The model under review builds one solid part; all positions refer to its coordinate system, in mm. A direction names the side the tool comes from. Coordinates: 2 decimals unless noted, no trailing zeros. Loops run counter-clockwise (first coordinate to the right, second up) from the corner with the lowest first, then second, coordinate; pieces in that order, holes last. Notation, with made-up numbers: M 15.5,-24.75 L 25.5,-24.75 A25 ccw 25.5,12.25 Z; hole C 62,-19 d10. An arc over 180 degrees is marked long. One line per item, written item: value.
```python
from build123d import *

# Parameters (mm, degrees)
SKICA2_W                 = 95
SKICA2_H                 = 50
SKICA2_W_2               = 92.6
SKICA2_H_2               = 47.6
P_IDAT_VYSUNUT_M3_DEPTH  = 11
SKICA7_R                 = 1.2
SKICA7_W                 = 11
SKICA7_H                 = 6.3
ODEBRAT_VYSUNUT_M1_DEPTH = 71.924466864
SKICA8_R                 = 2.65
SKICA8_W                 = 15.4
SKICA8_H                 = 7.7
ODEBRAT_VYSUNUT_M2_DEPTH = 71.924466864
SKICA9_R                 = 3.15
ODEBRAT_VYSUNUT_M3_DEPTH = 15
SKICA12_W                = 95
SKICA12_H                = 50
P_IDAT_VYSUNUT_M4_DEPTH  = 1.2
SKICA13_R                = 8
SKICA13_W                = 22
SKICA13_H                = 25
SKICA13_R_2              = 1.2
SKICA13_R_3              = 1.25
ODEBRAT_VYSUNUT_M4_DEPTH = 1.2


with BuildPart() as part:
    # Skica2 → Přidat vysunutím3 (new body)
    with BuildSketch(Plane.XY.offset(1.2)):
        with Locations((47.5, -25)):
            Rectangle(SKICA2_W, SKICA2_H)
        with Locations((47.5, -25)):
            Rectangle(SKICA2_W_2, SKICA2_H_2, mode=Mode.SUBTRACT)
    extrude(amount=P_IDAT_VYSUNUT_M3_DEPTH)

    # Skica7 → Odebrat vysunutím1 (cut, through all)
    with BuildSketch(Plane(origin=(45, -1.2, 0), x_dir=(1, 0, 0), z_dir=(0, -1, 0))):
        with Locations(Location((-20.9, 6.35, 0), (0, 0, 270))):
            Circle(SKICA7_R)
        with Locations(Location((-5.7, 6.35, 0), (0, 0, 270))):
            Circle(SKICA7_R)
        with Locations((-13.3, 6.35)):
            Rectangle(SKICA7_W, SKICA7_H)
    extrude(amount=-ODEBRAT_VYSUNUT_M1_DEPTH, mode=Mode.SUBTRACT)

    # Skica8 → Odebrat vysunutím2 (cut, through all)
    with BuildSketch(Plane(origin=(45, -1.2, 0), x_dir=(1, 0, 0), z_dir=(0, -1, 0))):
        with Locations(Location((2.2, 6.35, 0), (0, 0, 270))):
            Circle(SKICA8_R)
        with Locations(Location((10.2, 6.35, 0), (0, 0, 270))):
            Circle(SKICA8_R)
        with Locations((25.9, 6.35)):
            Rectangle(SKICA8_W, SKICA8_H)
    extrude(amount=-ODEBRAT_VYSUNUT_M2_DEPTH, mode=Mode.SUBTRACT)

    # Skica9 → Odebrat vysunutím3 (cut)
    with BuildSketch(Plane(origin=(45, -50, 0), x_dir=(1, 0, 0), z_dir=(0, -1, 0))):
        with Locations(Location((-20, 6.7, 0), (0, 0, 270))):
            Circle(SKICA9_R)
        with Locations(Location((-5, 6.7, 0), (0, 0, 270))):
            Circle(SKICA9_R)
        with Locations(Location((10, 6.7, 0), (0, 0, 270))):
            Circle(SKICA9_R)
        with Locations(Location((25, 6.7, 0), (0, 0, 270))):
            Circle(SKICA9_R)
        with Locations(Location((40, 6.7, 0), (0, 0, 270))):
            Circle(SKICA9_R)
        with Locations(Location((-35, 6.7, 0), (0, 0, 270))):
            Circle(SKICA9_R)
    extrude(amount=-ODEBRAT_VYSUNUT_M3_DEPTH, mode=Mode.SUBTRACT)

    # Skica12 → Přidat vysunutím4 (add)
    with BuildSketch(Plane(origin=(0, 0, 1.2), x_dir=(-1, 0, 0), z_dir=(0, 0, -1))):
        with Locations((-47.5, -25)):
            Rectangle(SKICA12_W, SKICA12_H)
    extrude(amount=P_IDAT_VYSUNUT_M4_DEPTH)

    # Skica13 → Odebrat vysunutím4 (cut)
    with BuildSketch(Plane.XY.offset(1.2)):
        with Locations((11.2, -11.2)):
            Circle(SKICA13_R)
        with Locations((70.8, -13.7)):
            Rectangle(SKICA13_W, SKICA13_H)
        with Locations((3.7, -3.7)):
            Circle(SKICA13_R_2)
        with Locations((91.3, -3.7)):
            Circle(SKICA13_R_3)
        with Locations((91.3, -46.3)):
            Circle(SKICA13_R_3)
        with Locations((3.7, -46.3)):
            Circle(SKICA13_R_3)
    extrude(amount=-ODEBRAT_VYSUNUT_M4_DEPTH, mode=Mode.SUBTRACT)


solid = part.part
```
(1) To check wall thickness, follow L1, parallel to Y at x = 91.3, z = 0.4; L2, parallel to Y at x = 50.5, z = 10.25; L3, parallel to X at y = -43.5, z = 10. State the ranges of each line that lie inside material, in increasing order. Write a range as [from, to].
Checks:
L1: [-50, -47.55], [-45.05, -4.95], [-2.45, 0]
L2: [-50, -48.8], [-1.2, 0]
L3: [0, 1.2], [93.8, 95]
(2) Add section D-D on y = -37. State the section outline as (x, z) points.
Checks:
outline: M 0,0 L 95,0 L 95,12.2 L 93.8,12.2 L 93.8,1.2 L 1.2,1.2 L 1.2,12.2 L 0,12.2 Z
(3) Tool access review of faces 5 (the face through (25.138, -49.408, 9.847)), 6 (the face through (18.83, -8.8, 0.61)), 7 (the face through (48, -25, 1.2)): name each direction out of +Z, -Z, +X, -X, +Y, -Y from which nothing blocks a thin tool from reaching the whole face with its end or side.
Checks:
face 5: -Y
face 6: +Z, -Z
face 7: +Z
(4) Add section A-A on x = 85. State the section outline as (y, z) points.
Checks:
outline: M -50,0 L 0,0 L 0,12.2 L -1.2,12.2 L -1.2,1.2 L -48.8,1.2 L -48.8,3.55 L -50,3.55 Z; M -50,9.85 L -48.8,9.85 L -48.8,12.2 L -50,12.2 Z
(5) Insertion check: pin 1 Ø3.5 at (y, z) = (-31.5, 5.5) entering from -X; pin 2 Ø1 at (x, y) = (42, -25.5) entering from +Z; pin 3 Ø3 at (x, z) = (39.3, 6.35) entering from -Y. Each pin has a flat end and moves straight along its axis. Give the tip position at first contact, or say it passes through.
Checks:
pin 1: x = 0
pin 2: z = 1.2
pin 3: y = -1.2
(6) Add section C-C on x = 70. State the section outline as (y, z) points.
Checks:
outline: M -50,0 L -26.2,0 L -26.2,1.2 L -48.8,1.2 L -48.8,3.55 L -50,3.55 Z; M -50,9.85 L -48.8,9.85 L -48.8,12.2 L -50,12.2 Z; M -1.2,0 L 0,0 L 0,2.5 L -1.2,2.5 Z; M -1.2,10.2 L 0,10.2 L 0,12.2 L -1.2,12.2 Z
(7) Draft analysis for pull direction Z (two halves, no side actions). For faces 1 (the face through (36.925, -49.408, 7.383)), 2 (the face through (47, -49, 12.2)), 3 (the face through (92.49, -3.32, 0.61)), 4 (the face through (49.83, -0.61, 6.69)), state which applies: pulls with the +Z half, pulls with the -Z half, needs draft (parallel to the pull), parting line crosses it, or undercut.
Checks:
face 1: undercut
face 2: pulls with the +Z half
face 3: needs draft
face 4: undercut
(8) Add section B-B on y = -46.3. State the section outline as (x, z) points.
Checks:
outline: M 0,0 L 2.45,0 L 2.45,1.2 L 1.2,1.2 L 1.2,12.2 L 0,12.2 Z; M 4.95,0 L 90.05,0 L 90.05,1.2 L 4.95,1.2 Z; M 92.55,0 L 95,0 L 95,12.2 L 93.8,12.2 L 93.8,1.2 L 92.55,1.2 Z
